Geometry: see drawing. Coordinates: mm, zero at the bounding-box minimum. Coordinates: 2 decimals unless noted, no trailing zeros. Order: outer loops, then holes, each group sorted by start corner. A loop starts at its lowest first (then second) coordinate and runs counter-clockwise, first axis right, second up. Notation, with made-up numbers: M -40,56.5 L 0,56.5 A27 ccw 0,78.5 Z; hole C 28,-18.75 d5. An arc over 180 degrees is marked long. One line per item, written item: value.
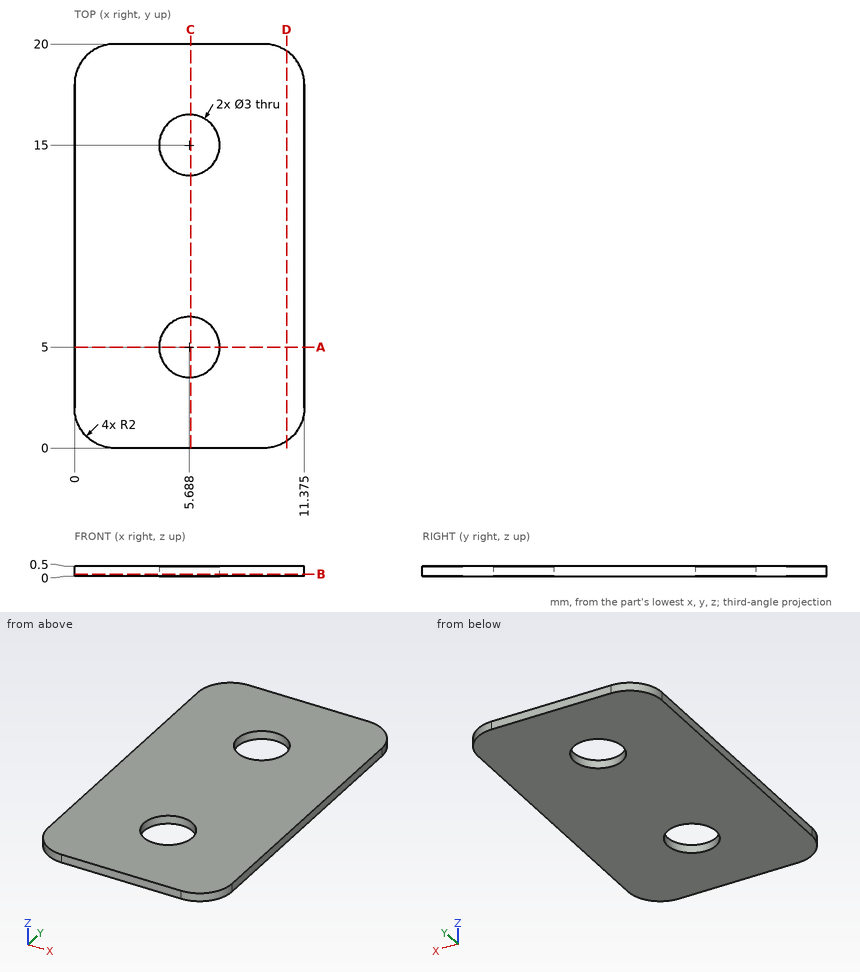
(1) Cut plane C-C on x = 5.75. Output: boundary loops of the cut face in (y, z).
Data:
outline: M 0,0 L 3.5,0 L 3.5,0.5 L 0,0.5 Z; M 6.5,0 L 13.5,0 L 13.5,0.5 L 6.5,0.5 Z; M 16.5,0 L 20,0 L 20,0.5 L 16.5,0.5 Z
(2) Cut plane B-B on z = 0.1. Output: boundary loops of the cut face in (x, y) (1 decimal).
Data:
outline: M 0,2 A2 ccw 2,0 L 9.4,0 A2 ccw 11.4,2 L 11.4,18 A2 ccw 9.4,20 L 2,20 A2 ccw 0,18 Z; hole C 5.7,5 d3; hole C 5.7,15 d3
(3) Ray query, line 1 (Y direction, x = 5.75, z = 0.25); line 2 (Y direction, x = 6.75, z = 0.35); line 3 (X direction, y = 15.5, z = 0.35) (1 decimal). Return the intervals inside material, ascending. Write a range as from..to.
Data:
line 1: y = 0..3.5, 6.5..13.5, 16.5..20
line 2: y = 0..3.94, 6.06..13.94, 16.06..20
line 3: x = 0..4.3, 7.1..11.4
(4) Cut plane D-D on x = 10.5. Output: boundary loops of the cut face in (y, z).
Data:
outline: M 0.35,0 L 19.65,0 L 19.65,0.5 L 0.35,0.5 Z
(5) Cut plane A-A on y = 5. Output: boundary loops of the cut face in (x, z) (1 decimal).
Data:
outline: M 0,0 L 4.2,0 L 4.2,0.5 L 0,0.5 Z; M 7.2,0 L 11.4,0 L 11.4,0.5 L 7.2,0.5 Z
